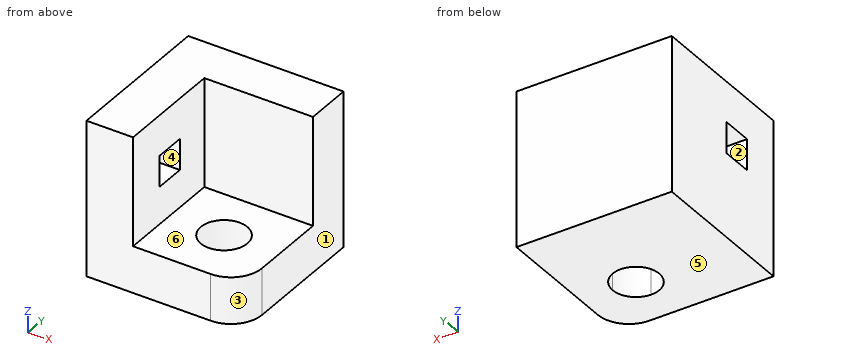
from build123d import *

# Parameters (mm, degrees)
F0_W      = 1270
F0_H      = 1270
F1_DEPTH  = 1270
F2_W      = 889
F2_H      = 889
F3_DEPTH  = 889
F4_W      = 254
F4_H      = 254
F5_DEPTH  = 381
F5_FACE_W = 254
F5_FACE_H = 254
F6_DEPTH  = 762
F8_DEPTH  = 381
F9_R      = 254


with BuildPart() as f1:
    # F0 (on Front) → F1 (new body)
    with BuildSketch(Plane.XZ):
        Rectangle(F0_W, F0_H)
    extrude(amount=F1_DEPTH)

    # F2 (on face) → F3 (cut)
    with BuildSketch(Plane.XZ.offset(1270)):
        with Locations((190.5, 190.5)):
            Rectangle(F2_W, F2_H)
    extrude(amount=-F3_DEPTH, mode=Mode.SUBTRACT)

    # F4 (on face) → F5 (join)
    with BuildSketch(Plane.YZ.offset(-254)):
        with Locations((-812.8, 177.8)):
            Rectangle(F4_W, F4_H)
    extrude(amount=F5_DEPTH)

    # F5_face (on face) → F6 (cut)
    with BuildSketch(Plane(origin=(127, -812.8, 177.8), x_dir=(0, 1, 0), z_dir=(1, 0, 0))):
        Rectangle(F5_FACE_W, F5_FACE_H)
    extrude(amount=-F6_DEPTH, mode=Mode.SUBTRACT)

    # F7 (on face) → F8 (cut)
    with BuildSketch(Plane.XY.offset(-254)):
        with BuildLine():
            ThreePointArc((381, -812.8), (55.796158, -678.096158), (190.5, -1003.3))
            ThreePointArc((190.5, -1003.3), (325.203842, -947.503842), (381, -812.8))
        make_face()
    extrude(amount=-F8_DEPTH, mode=Mode.SUBTRACT)

    # F9
    f9_edges = [f1.edges().sort_by_distance(p)[0] for p in [
        (635, -1270, -444.5),
    ]]
    fillet(f9_edges, radius=F9_R)


solid = f1.part
Geometry: final body of the model. Coordinates: model frame, mm. Face numbers are marked on the shaded views. A direction names the side the tool comes from. Give positions to 0.01 mm unless a question says otherwise; leave off trailing zeros. Write each loop counter-clockwise with the first axis right and the second up, starting at its lowest first coordinate (ties: lowest second). Pieces come first, ordered by that corner, then holes. Notation, with made-up numbers: (60, 88) - (106, 88) arc R33 cw to (106, 126) - close; hole circle Ø10 at (79, 17.25). An arc over 180 degrees is marked (long way). Return JSON: item names as keys, results as strings. Group by question number.
1) Line query: line 1 (Z direction, x = -298.5, y = -934); line 2 (X direction, y = -812, z = -418); line 3 (Y direction, x = 190, z = -483). Output: solid intervals per line, ascending.
2) First-contact query: P1, Ø10, axis at x = 163.5, z = 128, coming from the -Y side; P2, Ø1.5, axis at x = 460, z = 249, coming from the +Y side. Flat tips, straight axial feed; report the tip coordinate or a pass-through.
3) Mould query, pull axis Y, two halves, no side actions, for the marked faces 1, 2 and 3. Classes: released by +Y, released by -Y, zero draft, split by the parting line, or undercut.
4) Section C-C on y = -976.5. Return the cut outline in (x, z).
5) Section B-B on y = -786. Return the cut outline in (x, z).
6) Set-up query: the marked faces 4, 5 and 6. Return all of +Z, -Z, +X, -X, +Y, -Y with unobstructed straight access to the full face (end or side cutting, diameter ignored); none if empty.
7) Section D-D on x = 437.5. Return the cut outline in (y, z), plus the area to 3 significant figures.
8) Section A-A on z = -307. Return the cut outline in (x, y).
Filled in:
{
 "1": {"line 1": "z = -635 to 50.8, 304.8 to 635", "line 2": "x = -635 to 0, 381 to 635", "line 3": "y = -1270 to -1003.3, -622.3 to 0"},
 "2": {"P1": "stops at y = -381", "P2": "stops at y = 0"},
 "3": {"face 1": "zero draft", "face 2": "undercut", "face 3": "released by -Y"},
 "4": {"outline": "(-635, -635) - (93.07, -635) - (93.07, -254) - (-254, -254) - (-254, 635) - (-635, 635) - close; (287.93, -635) - (635, -635) - (635, -254) - (287.93, -254) - close"},
 "5": {"outline": "(-635, -635) - (1.89, -635) - (1.89, -254) - (-254, -254) - (-254, 50.8) - (-635, 50.8) - close; (-635, 304.8) - (-254, 304.8) - (-254, 635) - (-635, 635) - close; (379.11, -635) - (635, -635) - (635, -254) - (379.11, -254) - close"},
 "6": {"face 4": "+X, -X", "face 5": "-Z, +X, -X, +Y, -Y", "face 6": "+Z, +X, -Y"},
 "7": {"outline": "(-1263.64, -635) - (0, -635) - (0, 635) - (-381, 635) - (-381, -254) - (-1263.64, -254) - close", "area": "820,000 mm^2"},
 "8": {"outline": "(-635, -1270) - (381, -1270) arc R254 ccw to (635, -1016) - (635, 0) - (-635, 0) - close; hole circle Ø381 at (190.5, -812.8)"}
}
